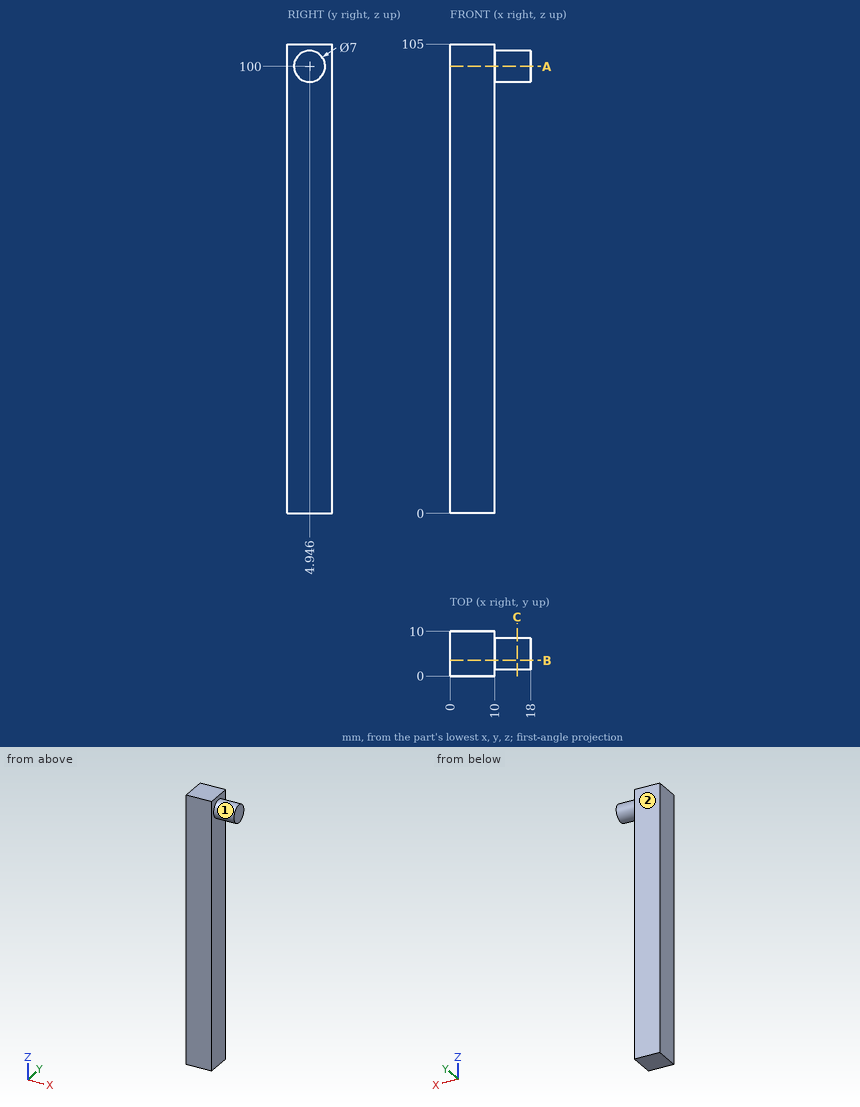
Geometry check sheet. Reference: drawing and pictorial views, mm from the part's lowest x, y, z. A direction names the side the tool comes from. Coordinates: 2 decimals unless noted, no trailing zeros. Order: outer loops, then holes, each group sorted by start corner. A loop starts at its lowest first (then second) coordinate and runs counter-clockwise, first axis right, second up. Notation, with made-up numbers: (-23, 67) -> (15, 67) arc R17 cw to (15, 98) -> close; hole circle Ø5 at (2, 31). An arc over 180 degrees is marked (long way). Write item = value, one per line. Start each with the question number.
1) Cross-section at A-A (z = 100). Enter the section's corners in (x, y).
2) Cross-section at B-B (y = 3.5). Enter the section's corners in (x, z).
3) Material ranges on L1, parallel to X at y = 8.25, z = 55; L2, parallel to Z at x = 11, y = 1.75; L3, parallel to Z at x = 15.5, y = 2.5, recorded low to high.
4) Access from +Z, -Z, +X, -X, +Y, -Y to the whole of each face (thin tool, end or side, straight path). Record for the marked faces 1 and 2.
5) Cross-section at C-C (x = 15). Enter the section's corners in (y, z), then the cut area to 3 significant figures.
6) Go/stop test with flat-tipped pins: P1, Ø3, axis at y = 3, z = 40, coming from the +X side; P2, Ø3, axis at x = 14, y = 6.5, coming from the -Z side. Record where each tip stops, or that it passes through.
Ans:
q1.outline = (0, 0) -> (10, 0) -> (10, 1.45) -> (18, 1.45) -> (18, 8.45) -> (10, 8.45) -> (10, 10) -> (0, 10) -> close
q2.outline = (0, 0) -> (10, 0) -> (10, 96.81) -> (18, 96.81) -> (18, 103.19) -> (10, 103.19) -> (10, 105) -> (0, 105) -> close
q3.L1 = 0 to 10
q3.L2 = 98.57 to 101.43
q3.L3 = 97.5 to 102.5
q4.face_1 = +X
q4.face_2 = +Z, -Z, +X, -X, +Y
q5.outline = circle Ø7 at (4.95, 100)
q5.area = 38.5 mm²
q6.P1 = 10
q6.P2 = 96.5
